Print and shaded views of the part. All mm, measured from the part's lowest x, y and z. Give positions to 0.01 mm unless a question says otherwise; leave off trailing zeros. Write each loop counter-clockwise with the first axis right and the second up, starting at its lowest first coordinate (ties: lowest second). Pieces come first, ordered by that corner, then holes. Notation, with made-up numbers: (-26.5, 56) -> (-12.5, 56) arc R30 ccw to (-12.5, 91) -> close; hole circle Ø5 at (39, 30.5). An arc over 180 degrees is marked (long way). Put each result on its own line as item: value.
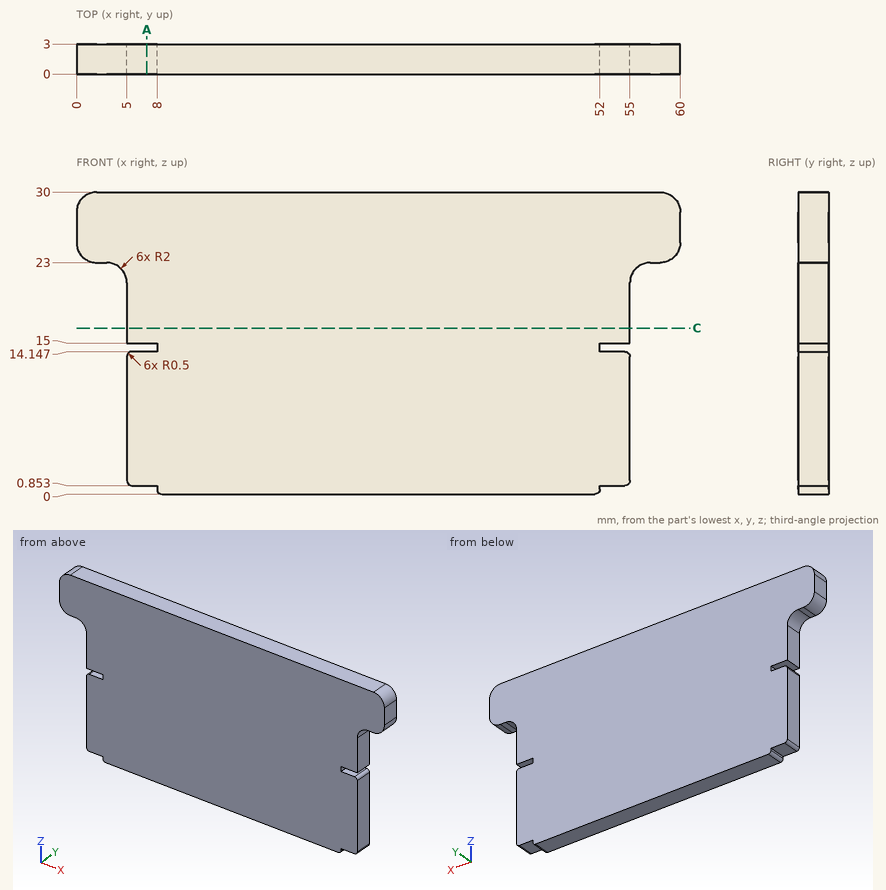
1) Slice it at A-A (x = 7). Write the cut outline in (y, z).
Filled sheet:
outline: (0, 0.85) -> (3, 0.85) -> (3, 14.15) -> (0, 14.15) -> close; (0, 15) -> (3, 15) -> (3, 30) -> (0, 30) -> close
2) Wall check: L1, parallel to Z at x = 54, y = 1.65; L2, parallel to X at y = 1.25, z = 18; L3, parallel to Z at x = 4.5, y = 1.15. Give the ranges that are in metal, low to high.
Filled sheet:
L1: 0.85 to 14.15, 15 to 30
L2: 5 to 55
L3: 22.32 to 30
3) Slice it at C-C (z = 16.5). Write the cut outline in (x, y).
Filled sheet:
outline: (5, 0) -> (55, 0) -> (55, 3) -> (5, 3) -> close
4) Pin check, flat tips, straight feed: pin 1 (1.5 mm diameter, centred on y = 1.5, z = 17, fed in from +X); pin 2 (1.5 mm diameter, centred on y = 1.5, z = 5.5, fed in from -X); pin 3 (1.2 mm diameter, centred on x = 6.5, y = 1.5, fed in from -Z). Stop position of each tip, or through.
Filled sheet:
pin 1: x = 55
pin 2: x = 5
pin 3: z = 0.85
